Verification items for the finished model (mm, model axes). Face numbers are marked on the shaded views. Give positions to 0.01 mm unless a question says otherwise; leave off trailing zeros. Write each loop counter-clockwise with the first axis right and the second up, starting at its lowest first coordinate (ties: lowest second). Pieces come first, ordered by that corner, then holes. Notation, with made-up numbers: (28, -22.5) - (69, -22.5) arc R15 ccw to (69, 0.5) - close; hole circle Ø2 at (49.5, 87). An arc over 180 degrees is marked (long way). Answer as a JSON object with one key per item and string values. Group by question number.
Item 1: Sectioned sample at C-C, the plane x = -26.5. Record the boundary of the cut face in (y, z) (1 decimal).
Item 2: Scan lines: line 1 along Y through (x, z) = (10, 0); line 2 along X through (y, z) = (-2, 4); line 3 along Y through (x, z) = (16.5, 2). Record each from-to range of solid material in increasing order. Write a range as [from, to].
Item 3: Sectioned sample at B-B, the plane z = 1. Record the boundary of the cut face in (x, y), and give its area (3 significant figures).
Item 4: Draft check along Z on the marked faces 1 and 2. Enter one of: +Z half, -Z half, draft (parallel to the pull), parting line (faces both ways), or undercut.
Item 5: Sectioned sample at A-A, the plane y = 0. Record the boundary of the cut face in (x, z), and give its area (3 significant figures).
Item 6: Go/stop test with flat-tipped pins: pin 1 (1.3 mm diameter, centred on x = 37, y = -4, fed in from +Z); pin 2 (2 mm diameter, centred on x = -5, y = 2, fed in from -Z); pin 3 (5 mm diameter, centred on y = -1, z = 2, fed in from +X). Record where each tip stops, or that it passes through.
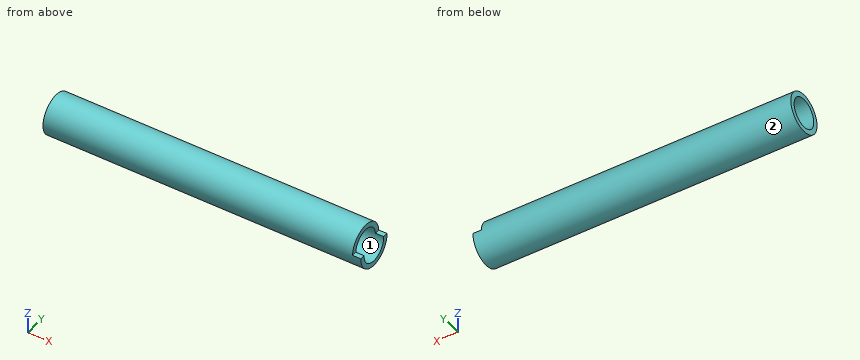
```python
from build123d import *

# Parameters (mm, degrees)
SKETCH3_R           = 4.7625
SKETCH3_R_2         = 3.571875
BOSS_EXTRUDE1_DEPTH = 38.1
SKETCH4_W           = 4
SKETCH4_H           = 11.464180208
CUT_EXTRUDE1_DEPTH  = 34.798


with BuildPart() as part:
    # Sketch3 → Boss-Extrude1 (new, symmetric)
    with BuildSketch(Plane(origin=(0, 0, 0), x_dir=(0, 0, -1), z_dir=(1, 0, 0))):
        with Locations(Location((0, 0, 0), (0, 0, 180))):
            Circle(SKETCH3_R)
        with Locations(Location((0, 0, 0), (0, 0, 180))):
            Circle(SKETCH3_R_2, mode=Mode.SUBTRACT)
    extrude(amount=BOSS_EXTRUDE1_DEPTH, both=True)

    # Sketch4 → Cut-Extrude1 (cut)
    with BuildSketch(Plane.XY.offset(35)):
        with Locations((38.1, 0)):
            Rectangle(SKETCH4_W, SKETCH4_H)
    extrude(amount=-CUT_EXTRUDE1_DEPTH, mode=Mode.SUBTRACT)


solid = part.part
```
Geometry check:
{
 "1": {"outline": "circle Ø9.5 at (0, 0); hole circle Ø7.1 at (0, 0)"},
 "2": {"line 1": "[-4.76, -3.57], [3.57, 4.76]", "line 2": "[-38.1, 36.1]", "line 3": "[-4.32, -2.96], [2.96, 4.32]"},
 "3": {"outline": "(-38.1, -4.66) - (36.1, -4.66) - (36.1, -3.43) - (-38.1, -3.43) - close; (-38.1, 3.43) - (36.1, 3.43) - (36.1, 4.66) - (-38.1, 4.66) - close", "area": "182 mm^2"},
 "4": {"face 1": "undercut", "face 2": "parting line"},
 "5": {"outline": "(-38.1, -4.76) - (38.1, -4.76) - (38.1, -3.57) - (-38.1, -3.57) - close; (-38.1, 3.57) - (36.1, 3.57) - (36.1, 4.76) - (-38.1, 4.76) - close", "area": "179 mm^2"},
 "6": {"pin 1": "z = 0.2", "pin 2": "z = -4.66", "pin 3": "x = 36.1"}
}
